Check sheet for the drawn part. Datum: minimum x, y, z corner. Units: mm. Round coordinates to 2 decimals unless told otherwise and drop trailing zeros. Order: outer loops, then holes, each group sorted by start corner. A loop starts at its lowest first (then second) coordinate and runs counter-clockwise, first axis right, second up. Notation, with made-up numbers: M 60,70 L 69,70 A26 ccw 69,97 Z; hole C -9,19.25 d4. An arc over 180 degrees is marked long. Answer as a JSON object with one key per item and string values. Group by question number.
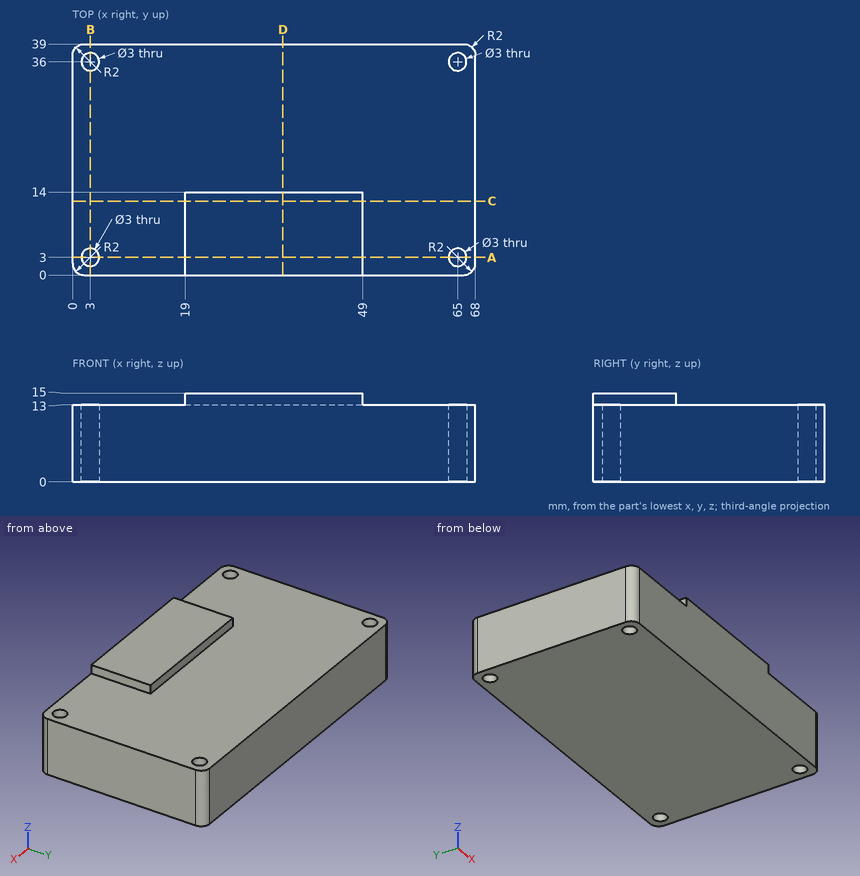
1) Thickness scan on line 1 along X through (y, z) = (36, 5.5); line 2 along Y through (x, z) = (65, 3.75); line 3 along Z through (x, y) = (13, 6.5). Record the ranges inside material, lowest first. Write a range as [from, to].
2) Sectioned sample at B-B (x = 3). Record the boundary of the cut face in (y, z), then the cut area to 3 significant figures.
3) Sectioned sample at A-A (y = 3). Record the boundary of the cut face in (x, z).
4) Sectioned sample at C-C (y = 12.5). Record the boundary of the cut face in (x, z), then the cut area to 3 significant figures.
5) Go/stop test with flat-tipped pins: P1, Ø1.6, axis at y = 8.5, z = 14, coming from the -X side; P2, Ø2, axis at x = 46.5, y = 34.5, coming from the +Z side; P3, Ø0.6, axis at x = 30, z = 14, coming from the +Y side. Record where each tip stops, or that it passes through.
6) Sectioned sample at D-D (x = 35.5). Record the boundary of the cut face in (y, z).
Final values:
{
 "1": {"line 1": "x = [0, 1.5], [4.5, 63.5], [66.5, 68]", "line 2": "y = [0, 1.5], [4.5, 34.5], [37.5, 39]", "line 3": "z = [0, 13]"},
 "2": {"outline": "M 0,0 L 1.5,0 L 1.5,13 L 0,13 Z; M 4.5,0 L 34.5,0 L 34.5,13 L 4.5,13 Z; M 37.5,0 L 39,0 L 39,13 L 37.5,13 Z", "area": "429 mm^2"},
 "3": {"outline": "M 0,0 L 1.5,0 L 1.5,13 L 0,13 Z; M 4.5,0 L 63.5,0 L 63.5,13 L 49,13 L 49,15 L 19,15 L 19,13 L 4.5,13 Z; M 66.5,0 L 68,0 L 68,13 L 66.5,13 Z"},
 "4": {"outline": "M 0,0 L 68,0 L 68,13 L 49,13 L 49,15 L 19,15 L 19,13 L 0,13 Z", "area": "944 mm^2"},
 "5": {"P1": "stops at x = 19", "P2": "stops at z = 13", "P3": "stops at y = 14"},
 "6": {"outline": "M 0,0 L 39,0 L 39,13 L 14,13 L 14,15 L 0,15 Z"}
}
